CAD build for the part. Positions are in the model's coordinates, mm. A direction names the side the tool comes from. Round coordinates to 2 decimals unless told otherwise and drop trailing zeros. Order: outer loops, then holes, each group sorted by start corner. A loop starts at its lowest first (then second) coordinate and runs counter-clockwise, first axis right, second up. Notation, with made-up numbers: M 12.5,37 L 22.5,37 A29 cw 22.5,59 Z; hole C 59,-7.5 d1. An arc over 180 degrees is marked long. Answer as a JSON object with one key per item and string values. Group by question number.
Autodesk Inventor part; units mm, degrees
ref_plane "YZ Plane" through (0, 0, 0) normal (1, 0, 0) x (0, 1, 0)
ref_plane "XZ Plane" through (0, 0, 0) normal (0, 1, 0) x (-1, 0, 0)
ref_plane "XY Plane" through (0, 0, 0) normal (0, 0, 1) x (1, 0, 0)
sketch "Sketch1" plane through (0, 0, 0) normal (0, 1, 0) x (-1, 0, 0)
  line L0 (0, 0) -> (-335, 0)
  line L1 (-335, 0) -> (-335, -15)
  line L2 (-335, -15) -> (0, -15)
  line L3 (0, -15) -> (0, 0)
  dimension "d0" = 15
  dimension "d1" = 335
extrude "Extrusion1" add sketch "Sketch1" along normal blind 6.5
sketch "Sketch2" plane through (0, 6.5, 0) normal (0, 1, 0) x (1, 0, 0)
  line L0 (0, 0) -> (335, 0)
  line L1 (335, 0) -> (335, 15)
  line L2 (0, 15) -> (0, 0)
  line L3 (0, 12) -> (-4.5, 12)
  line L4 (-6.5, 10) -> (-6.5, 6)
  line L5 (-4.5, 4) -> (0, 4)
  line L6 (0, 4) -> (0, 12)
  line L7 (335, 12) -> (339.5, 12)
  line L8 (341.5, 10) -> (341.5, 6)
  line L9 (339.5, 4) -> (335, 4)
  line L10 (335, 4) -> (335, 12)
  line L11 (80, 0) -> (88, 0)
  line L12 (88, 0) -> (88, -4.5)
  line L13 (86, -6.5) -> (82, -6.5)
  line L14 (80, -4.5) -> (80, 0)
  line L15 (247, 0) -> (255, 0)
  line L16 (255, 0) -> (255, -4.5)
  line L17 (253, -6.5) -> (249, -6.5)
  line L18 (247, -4.5) -> (247, 0)
  arc A0 (-4.5, 12) -> (-6.5, 10) centre (-4.5, 10) ccw
  arc A1 (-6.5, 6) -> (-4.5, 4) centre (-4.5, 6) ccw
  arc A2 (80, -4.5) -> (82, -6.5) centre (82, -4.5) ccw
  arc A3 (86, -6.5) -> (88, -4.5) centre (86, -4.5) ccw
  arc A4 (247, -4.5) -> (249, -6.5) centre (249, -4.5) ccw
  arc A5 (253, -6.5) -> (255, -4.5) centre (253, -4.5) ccw
  arc A6 (339.5, 4) -> (341.5, 6) centre (339.5, 6) ccw
  arc A7 (341.5, 10) -> (339.5, 12) centre (339.5, 10) ccw
  dimension "d4" = 2
  dimension "d5" = 8
  dimension "d6" = 8
  dimension "d7" = 8
  dimension "d8" = 8
  dimension "d9" = 6.5
  dimension "d10" = 6.5
  dimension "d11" = 6.5
  dimension "d12" = 4
  dimension "d13" = 80
  dimension "d14" = 80
extrude "Extrusion2" add sketch "Sketch2" against normal blind 6.5
equation "\"d6\" = d5"
equation "\"d7\" = d6"
equation "\"d8\" = d7"
equation "\"d10\" = d9"
equation "\"d11\" = d9"
equation "\"d14\" = d13"
properties part number "front_upper_brace"
Item 1: Drill centre lines: line 1 (X direction, y = 1, z = 0.25); line 2 (X direction, y = 4.75, z = -12.75); line 3 (Z direction, x = 256.5, y = 5.5). Where is each one in solid material? Low to high. Write a range as [from, to].
Item 2: Cut at B-B, the plane x = 306. Give the cut face in (y, z), and give its area (3 significant figures).
Item 3: 3-axis set-ups, long thin cutter, end or side, ignore diameter. For faces 4 (the face through (166, 3, 0)), 5 (the face through (294, 3, 0)), 6 (the face through (170, 3, -15)): which of +Z, -Z, +X, -X, +Y, -Y reach the whole face in a straight line?
Item 4: Cut at A-A, the plane y = 3.5. Give the cut face in (x, z), and give its area (3 significant figures).
Item 5: Flat gauge pins, fed straight in: pin 1 Ø2 at (x, y) = (-1.5, 3) entering from -Z; pin 2 Ø3 at (y, z) = (4.5, 4) entering from +X; pin 3 Ø3.5 at (x, y) = (-2.5, 2) entering from +Z. Where does each tip first touch, or does it go through?
Item 6: Two-plate mould, pull along Y, no slides. Class faces 1 (the face through (39, 3, 0)), 2 (the face through (170, 0, -6)), 3 (the face through (170, 6.5, -6)): +Y half, -Y half, draft (parallel to the pull), parting line (faces both ways), or undercut.
Response values:
{
 "1": {"line 1": "[80, 88], [247, 255]", "line 2": "[0, 335]", "line 3": "[-15, 0]"},
 "2": {"outline": "M 0,-15 L 6.5,-15 L 6.5,0 L 0,0 Z", "area": "97.5 mm^2"},
 "3": {"face 4": "+Z, +Y, -Y", "face 5": "+Z, +X, +Y, -Y", "face 6": "-Z, +X, -X, +Y, -Y"},
 "4": {"outline": "M -6.5,-10 A2 ccw -4.5,-12 L 0,-12 L 0,-15 L 335,-15 L 335,-12 L 339.5,-12 A2 ccw 341.5,-10 L 341.5,-6 A2 ccw 339.5,-4 L 335,-4 L 335,0 L 255,0 L 255,4.5 A2 ccw 253,6.5 L 249,6.5 A2 ccw 247,4.5 L 247,0 L 88,0 L 88,4.5 A2 ccw 86,6.5 L 82,6.5 A2 ccw 80,4.5 L 80,0 L 0,0 L 0,-4 L -4.5,-4 A2 ccw -6.5,-6 Z", "area": "5,230 mm^2"},
 "5": {"pin 1": "z = -12", "pin 2": "x = 255", "pin 3": "z = -4"},
 "6": {"face 1": "draft", "face 2": "-Y half", "face 3": "+Y half"}
}
